```python
from build123d import *

# Parameters (mm, degrees)
SKETCH006_AS_DRAWN_W                 = 85
SKETCH006_AS_DRAWN_H                 = 40
EXTRUDE002_DEPTH                     = 80
EXTRUDE002_ONTO_SKETCH006_ROLL_ANGLE = 90
SKETCH005_R                          = 39.095168
EXTRUDE001_DEPTH                     = 60
EXTRUDE_DEPTH                        = 5
SKETCH004_W                          = 93
SKETCH004_H                          = 50
PAD_DEPTH                            = 20
REVOLUTION_ANGLE                     = -180


with BuildPart() as extrude002:
    # Sketch006 as drawn → Extrude002 (new)
    with BuildSketch(Plane.XY):
        with Locations((0, 25)):
            Rectangle(SKETCH006_AS_DRAWN_W, SKETCH006_AS_DRAWN_H)
    extrude(amount=EXTRUDE002_DEPTH)


with BuildPart() as extrude002_1:
    # Extrude002 onto Sketch006 roll: moved
    add(extrude002.part.rotate(Axis((0, 0, 0), (1, 0, 0)), EXTRUDE002_ONTO_SKETCH006_ROLL_ANGLE))


with BuildPart() as extrude002_2:
    # Extrude002 onto Sketch006 placement: moved
    add(extrude002_1.part.moved(Location((0, -27.5, 0))))


with BuildPart() as extrude001:
    # Sketch005 → Extrude001 (new body)
    with BuildSketch(Plane(origin=(0, 0, 0), x_dir=(1, 0, 0), z_dir=(0, 0, -1))):
        Circle(SKETCH005_R)
    extrude(amount=-EXTRUDE001_DEPTH)


with BuildPart() as cut:
    # Sketch003 → Extrude (new body)
    with BuildSketch(Plane(origin=(-42.5, -27.5, 45), x_dir=(0, 0, 1), z_dir=(0, 1, 0))):
        Polygon((0, 64), (5, 64), (5, 89), (-45, 89), (-45, 64), (-40, 64), (-40, 85), (0, 85), align=None)
        Polygon((0, 21), (5, 21), (5, -4), (-45, -4), (-45, 21), (-40, 21), (-40, 0), (0, 0), align=None)
    extrude(amount=-EXTRUDE_DEPTH)

    # Sketch004 → Pad (new body)
    with BuildSketch(Plane(origin=(0, -27.5, 0), x_dir=(-1, 0, 0), z_dir=(0, 1, 0))):
        with Locations((0, 25)):
            Rectangle(SKETCH004_W, SKETCH004_H)
    extrude(amount=PAD_DEPTH)

    # Cut: cut Extrude001
    add(extrude001.part, mode=Mode.SUBTRACT)


with BuildPart() as cut001:
    # Sketch → Revolution (revolve)
    with BuildSketch(Plane.XZ):
        Polygon((32.5, 50), (15, 32.5), (15, 17.5), (32.5, 0), (47.5, 0), (47.5, 50), align=None)
    revolve(axis=Axis((0, 0, 0), (0, 0, 1)), revolution_arc=REVOLUTION_ANGLE)

    # Fusion: union Cut
    add(cut.part)

    # Cut001: cut Extrude002
    add(extrude002_2.part, mode=Mode.SUBTRACT)


solid = cut001.part
```
Build history of the part. All positions in model axes, mm. A direction names the side the tool comes from. Round coordinates to 2 decimals unless told otherwise and drop trailing zeros. Write each loop counter-clockwise with the first axis right and the second up, starting at its lowest first coordinate (ties: lowest second). Pieces come first, ordered by that corner, then holes.
1) 3-axis set-ups, long thin cutter, end or side, ignore diameter. For faces 4 (the cylindrical face through (0, -15, 25)), 5 (the conical face through (0.434, -19.734, 37.239)), 6 (the flat face through (-43, -32.5, 25)), 7 (the flat face through (46.5, -21, 25)), 8 (the flat face through (-42.5, -30, 25)): which of +Z, -Z, +X, -X, +Y, -Y reach the whole face in a straight line?
2) Drill centre lines: probe 1 along X at (y, z) = (-30, 27.5); probe 2 along Z at (x, y) = (8, -31.5); probe 3 along X at (y, z) = (-19, 30.5). Where is each one in solid material? Low to high.
3) Mould opens along Z. For faces 1 (the flat face through (1, -35, 0)), 2 (the flat face through (-35, 0, 25)), 3 (the flat face through (42.5, -30, 25)) say: +Z half, -Z half, draft (parallel to the pull), parting line (faces both ways), or undercut.
4) Pin check, flat tips, straight feed: pin 1 (1 mm diameter, centred on y = -6.5, z = 43, fed in from +X); pin 2 (2 mm diameter, centred on x = 30, z = 34, fed in from -Y); pin 3 (25 mm diameter, centred on y = -24.5, z = 18, fed in from +X). Stop position of each tip, or through.
5) Band-saw the part on A-A, the plane z = 23. List the corners of the cut face in (x, y), and give its area (3 significant figures).
Ans:
1. face 4: +Z, -Z, +Y
1. face 5: +Z, +Y
1. face 6: +Z, -Z, -X, -Y
1. face 7: +Z, -Z, +X, -Y
1. face 8: -Y
2. probe 1: x = -46.5 to -42.5, 42.5 to 46.5
2. probe 2: z = 0 to 5, 45 to 50
2. probe 3: x = -46.5 to 46.5
3. face 1: -Z half
3. face 2: draft
3. face 3: undercut
4. pin 1: stops at x = 47.12
4. pin 2: stops at y = -27.5
4. pin 3: stops at x = 46.5
5. outline: (-47.5, 0) arc R47.5 ccw to (-46.5, -9.7) - (-46.5, -32.5) - (-42.5, -32.5) - (-42.5, -27.5) - (42.5, -27.5) - (42.5, -32.5) - (46.5, -32.5) - (46.5, -9.7) arc R47.5 ccw to (47.5, 0) - (15, 0) arc R15 cw to (-15, 0) - close
5. area: 2,260 mm2
